Read the model definition and answer for the solid it produces. Units are mm, in the model's axes. A direction names the side the tool comes from. Give positions to 0.01 mm unless a question says otherwise; leave off trailing zeros. Loops run counter-clockwise (first coordinate to the right, second up) from the corner with the lowest first, then second, coordinate; pieces in that order, holes last.
(1) Each of these flat-tipped pins is pushed along its axis until it touches: P1, Ø1.9, axis at y = 6, z = 0.5, coming from the -X side; P2, Ø4, axis at x = 0, z = 0, coming from the -Y side; P3, Ø3.5, axis at x = -10.5, y = 4.5, coming from the +Z side; P4, Ø3.5, axis at x = -11.5, y = 6.5, coming from the -Z side. Where does it stop, or does it pass through?
(2) Find section C-C, the plane x = 0. Write down the section's boundary in (y, z) (3 decimals), then the cut area to 3 significant figures.
(3) Which of the six approach directions +Z, -Z, +X, -X, +Y, -Y give full straight-line access (tool end or side, diameter ignored) to faces 1 (the face through (-11.47, 0.38, -4.4)), 2 (the face through (-12, 5, -4.762)), 3 (the face through (-6.248, 5, 0)), 4 (the face through (-11.678, 9.143, 4.4)), 5 (the face through (-11, 5, 4.762))?
(4) Straight lines are drawn through the part: probe 1 along Y at (x, z) = (-15.25, 0) (1 decimal); probe 2 along X at (y, z) = (5.75, 0) (3 decimals); probe 3 along X at (y, z) = (1.25, 2). For each, find the intervals that lie inside material, in ascending order.
(5) Determine the mould class of faces 6 (the face through (-12.687, 1.663, -0.688)), 7 (the face through (-6, 9.525, 0)), 8 (the face through (-0.69, 4.7, 3.1)) for opening direction Y: pulls with the +Y half, pulls with the -Y half, needs draft (parallel to the pull), parting line crosses it, or undercut.
```python
from build123d import *

# Parameters (mm, degrees)
SKETCH1_R           = 3.175
BOSS_EXTRUDE1_DEPTH = 9.525
FILLET1_R           = 1.27
SKETCH2_R           = 3.175
CUT_EXTRUDE1_DEPTH  = 12.7


with BuildPart() as part:
    # Sketch1 → Boss-Extrude1 (new body)
    with BuildSketch(Plane(origin=(0, 0, 0), x_dir=(1, 0, 0), z_dir=(0, 1, 0))):
        with BuildLine():
            Line((-4.200130206, -4.7625), (-18.948458917, -4.7625))
            Line((-18.948458917, -4.7625), (-18.948458917, 4.7625))
            Line((-18.948458917, 4.7625), (-4.200130206, 4.7625))
            ThreePointArc((-4.200130206, 4.7625), (6.35, 0), (-4.200130206, -4.7625))
        make_face()
        Circle(SKETCH1_R, mode=Mode.SUBTRACT)
    extrude(amount=BOSS_EXTRUDE1_DEPTH)

    # Fillet1
    fillet1_edges = [part.edges().sort_by_distance(p)[0] for p in [
        (-11.574294562, 9.525, -4.7625),
        (-11.574294562, 0, -4.7625),
        (-11.574294562, 0, 4.7625),
        (-11.574294562, 9.525, 4.7625),
    ]]
    fillet(fillet1_edges, radius=FILLET1_R)

    # Sketch2 → Cut-Extrude1 (cut)
    with BuildSketch(Plane.ZY.offset(18.948458917)):
        with Locations((0, 4.7625)):
            Circle(SKETCH2_R)
    extrude(amount=-CUT_EXTRUDE1_DEPTH, mode=Mode.SUBTRACT)


solid = part.part
```
Entries:
1. P1: stops at x = -6.25
1. P2: passes through
1. P3: stops at z = 4.76
1. P4: stops at z = -4.76
2. outline: (0, -6.35) - (9.525, -6.35) - (9.525, -3.175) - (0, -3.175) - close; (0, 3.175) - (9.525, 3.175) - (9.525, 6.35) - (0, 6.35) - close
2. area: 60.5 mm2
3. face 1: -Z, -X, -Y
3. face 2: -Z, -X, +Y, -Y
3. face 3: -X
3. face 4: +Z, -X, +Y
3. face 5: +Z, -X, +Y, -Y
4. probe 1: y = 0 to 1.6, 7.9 to 9.5
4. probe 2: x = -6.248 to -3.175, 3.175 to 6.35
4. probe 3: x = -18.95 to -2.47, 2.47 to 6.03
5. face 6: undercut
5. face 7: pulls with the +Y half
5. face 8: needs draft
